Design review of the part shown in the three views and the two pictorial views. Dimensions are in mm from the part's minimum x, y and z. Round coordinates to 2 decimals unless told otherwise and drop trailing zeros. Order: outer loops, then holes, each group sorted by start corner. A loop starts at its lowest first (then second) coordinate and runs counter-clockwise, first axis right, second up.
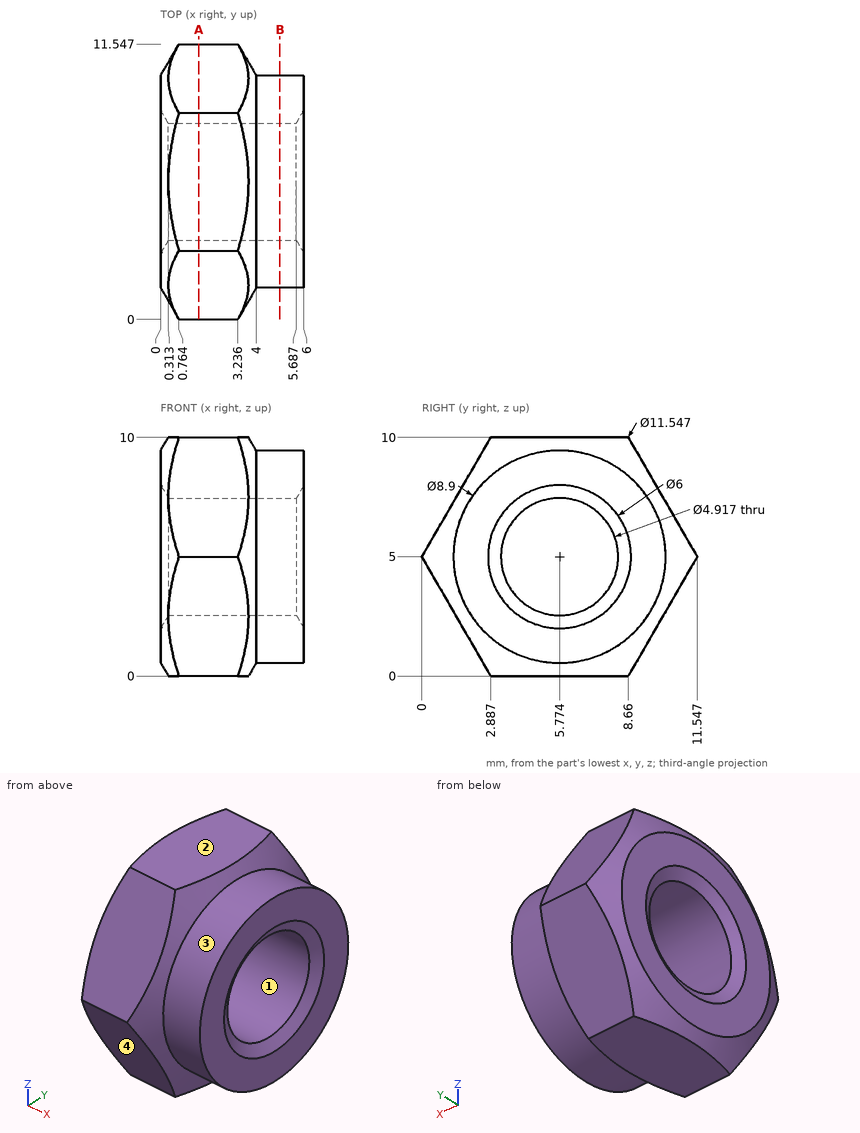
1) The part is to be moulded in two halves that separate along Z. For the marked faces 1, 2, 3 and 4, say which applies: released by +Z, released by -Z, zero draft, split by the parting line, or undercut.
Results:
face 1: undercut
face 2: released by +Z
face 3: split by the parting line
face 4: released by -Z
2) Take a section at B-B on x = 5. Give the boundary of the cut face in (y, z).
Results:
outline: circle Ø8.9 at (5.77, 5); hole circle Ø4.92 at (5.77, 5)
3) To check wall thickness, follow line 1 along Y through (x, z) = (4.45, 5) (1 decimal); line 2 along Z through (x, y) = (4.45, 6.5); line 3 along Y through (x, z) = (1.8, 5.5) (1 decimal). State the ranges of each line that lie inside material, in increasing order.
Results:
line 1: y = 1.3 to 3.3, 8.2 to 10.2
line 2: z = 0.61 to 2.65, 7.35 to 9.39
line 3: y = 0.3 to 3.4, 8.2 to 11.3
4) Take a section at A-A on x = 1.6. Give the boundary of the cut face in (y, z).
Results:
outline: (0, 5) - (2.89, 0) - (8.66, 0) - (11.55, 5) - (8.66, 10) - (2.89, 10) - close; hole circle Ø4.92 at (5.77, 5)
5) Clearance check with flat-ended pins moving along their axes: P1, Ø1.5, axis at x = 4, z = 7, coming from the +Y side (1 decimal); P2, Ø4, axis at y = 10, z = 1.5, coming from the +X side; P3, Ø4.5, axis at y = 5.77, z = 5, coming from the -X side. State where each tip first meets the part, or that it passes through.
Results:
P1: stops at y = 10.8
P2: stops at x = 6
P3: passes through
